```python
from build123d import *

# Parameters (mm, degrees)
SKETCH1_W           = 18
SKETCH1_H           = 50
BOSS_EXTRUDE1_DEPTH = 18


with BuildPart() as part:
    # Sketch1 → Boss-Extrude1 (new body)
    with BuildSketch(Plane.XY):
        Polygon((-300.514492677, 322.5), (299.485507323, 322.5), (299.485507323, 287.5), (316.971014646, 287.5), (316.971014646, 237.5), (299.485507323, 237.5), (299.485507323, -292.5), (318, -292.5), (318, -342.5), (299.485507323, -342.5), (299.485507323, -377.5), (174.485507323, -377.5), (174.485507323, -386.5), (124.485507323, -386.5), (124.485507323, -377.5), (-125.514492677, -377.5), (-125.514492677, -386.5), (-175.514492677, -386.5), (-175.514492677, -377.5), (-300.514492677, -377.5), (-300.514492677, -342.5), (-318, -342.5), (-318, -292.5), (-300.514492677, -292.5), (-300.514492677, 237.5), (-318, 237.5), (-318, 287.5), (-300.514492677, 287.5), align=None)
        with Locations((-150, 262.5)):
            Rectangle(SKETCH1_W, SKETCH1_H, mode=Mode.SUBTRACT)
        with Locations((0, 262.5)):
            Rectangle(SKETCH1_W, SKETCH1_H, mode=Mode.SUBTRACT)
        with Locations((0, 87.5)):
            Rectangle(SKETCH1_W, SKETCH1_H, mode=Mode.SUBTRACT)
    extrude(amount=BOSS_EXTRUDE1_DEPTH)


solid = part.part
```
The listing builds one solid part. Answer for the finished solid, in the listing's coordinates (mm). A direction names the side the tool comes from. Give positions to 0.01 mm unless a question says otherwise; leave off trailing zeros. Order: outer loops, then holes, each group sorted by start corner. A loop starts at its lowest first (then second) coordinate and runs counter-clockwise, first axis right, second up. Notation, with made-up numbers: (24.25, 55.5) -> (73.25, 55.5) arc R34 ccw to (73.25, 85.5) -> close; hole circle Ø9 at (56.25, 0.25). An arc over 180 degrees is marked (long way). Answer as a JSON object with one key per item and string values. Group by question number.
Item 1: The part is cut by section C-C on z = 4. Give the number of separate pieces and of enclosed holes in the cut face, and give its area (3 significant figures).
Item 2: The part is cut by section B-B on y = 84. Write down the section's boundary in (x, z).
Item 3: Determine the mould class of faces 5 (the flat face through (-159, 262, 9)), 6 (the flat face through (-309, 287.5, 9)), 7 (the flat face through (299.486, -360, 9)) for opening direction X: pulls with the +X half, pulls with the -X half, needs draft (parallel to the pull), parting line crosses it, or undercut.
Item 4: Consider L1, parallel to Y at x = 6, z = 12.75; L2, parallel to X at y = 64, z = 12.25; L3, parallel to X at y = 150.5, z = 13.75. Determine where each line is inside the solid, lowest interval first. Write a range as from..to.
Item 5: The part is cut by section A-A on y = 276.5. Write down the section's boundary in (x, z).
Item 6: A tool of negligible diameter and unlimited length cuts with its end or side. For faces 1 (the flat face through (308, 287.5, 9)), 2 (the flat face through (308, 237.5, 9)), 3 (the flat face through (-300.514, -360, 9)), 4 (the flat face through (0, 287.5, 9)), from which of +Z, -Z, +X, -X, +Y, -Y can it reach the whole face along a straight path? Write none if from no direction.
Item 7: Flat-ended cylindrical pins translate along their axes: pin 1 (3 mm diameter, centred on y = -198.5, z = 10, fed in from +X); pin 2 (9 mm diameter, centred on x = -18.5, z = 12.5, fed in from -Y); pin 3 (8.5 mm diameter, centred on x = -307, z = 10.5, fed in from -Y). Find the tip coordinate at first contact, or state that the pin passes through.
Item 8: The part is cut by section D-D on y = -132.5. Write down the section's boundary in (x, z), and give its area (3 significant figures).
Result set:
{
 "1": {"separate pieces": "1", "enclosed holes": "3", "area": "422,000 mm²"},
 "2": {"outline": "(-300.51, 0) -> (-9, 0) -> (-9, 18) -> (-300.51, 18) -> close; (9, 0) -> (299.49, 0) -> (299.49, 18) -> (9, 18) -> close"},
 "3": {"face 5": "undercut", "face 6": "needs draft", "face 7": "pulls with the +X half"},
 "4": {"L1": "-377.5..62.5, 112.5..237.5, 287.5..322.5", "L2": "-300.51..-9, 9..299.49", "L3": "-300.51..299.49"},
 "5": {"outline": "(-318, 0) -> (-159, 0) -> (-159, 18) -> (-318, 18) -> close; (-141, 0) -> (-9, 0) -> (-9, 18) -> (-141, 18) -> close; (9, 0) -> (316.97, 0) -> (316.97, 18) -> (9, 18) -> close"},
 "6": {"face 1": "+Z, -Z, +X, +Y", "face 2": "+Z, -Z, +X", "face 3": "+Z, -Z, -X, -Y", "face 4": "+Z, -Z"},
 "7": {"pin 1": "x = 299.49", "pin 2": "y = -377.5", "pin 3": "y = -342.5"},
 "8": {"outline": "(-300.51, 0) -> (299.49, 0) -> (299.49, 18) -> (-300.51, 18) -> close", "area": "10,800 mm²"}
}
